Drawing for the job (mm, zero at the part's lowest x, y, z). Give positions to 0.01 mm unless a question says otherwise; leave off trailing zeros. Loops run counter-clockwise (first coordinate to the right, second up) from the corner with the lowest first, then second, coordinate; pieces in that order, holes last. Notation, with made-up numbers: M 14.5,-39 L 54.5,-39 A16 ccw 54.5,-21 Z; hole C 77,12 d3. An arc over 180 degrees is marked long. Answer in a Markdown table with one row per item. Add a question column.
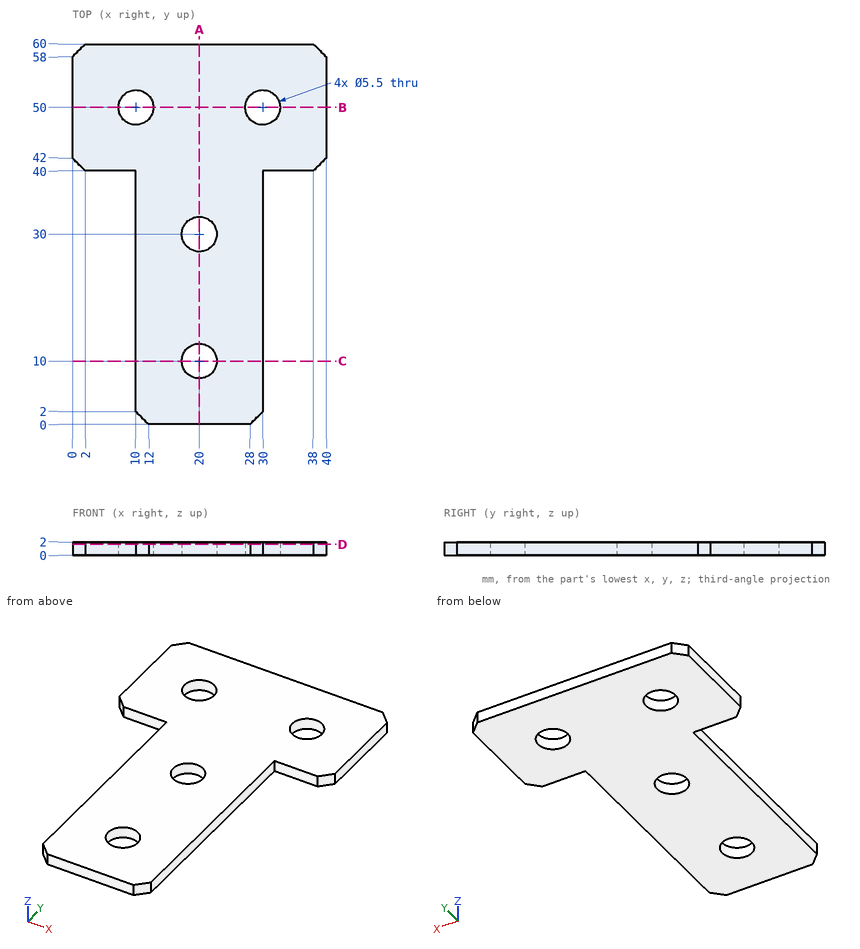
(1) Pin check, flat tips, straight feed: pin 1 (1 mm diameter, centred on x = 35, z = 0.5, fed in from -Y); pin 2 (1 mm diameter, centred on y = 14, z = 1, fed in from +X); pin 3 (3.5 mm diameter, centred on x = 30, y = 50, fed in from +Z); pin 4 (1 mm diameter, centred on x = 29, z = 1.5, fed in from -Y). Stop position of each tip, or through.
(2) Slice it at C-C, the plane y = 10. Give the cut face in (x, z), then the cut area to 3 significant figures.
(3) Slice it at B-B, the plane y = 50. Give the cut face in (x, z).
(4) Slice it at D-D, the plane z = 1.7. Give the cut face in (x, y).
(5) Wall check: line 1 (Y direction, x = 20, z = 1.55); line 2 (X direction, y = 51, z = 0.1); line 3 (X direction, y = 38, z = 0.45). Give the ranges that are in metal, low to high.
(6) Slice it at A-A, the plane x = 20. Give the cut face in (y, z), then the cut area to 3 significant figures.
Solution:
| question | item | result |
|---|---|---|
| 1 | pin 1 | y = 40 |
| 1 | pin 2 | x = 30 |
| 1 | pin 3 | through |
| 1 | pin 4 | y = 0.5 |
| 2 | outline | M 10,0 L 17.25,0 L 17.25,2 L 10,2 Z; M 22.75,0 L 30,0 L 30,2 L 22.75,2 Z |
| 2 | area | 29.0 mm^2 |
| 3 | outline | M 0,0 L 7.25,0 L 7.25,2 L 0,2 Z; M 12.75,0 L 27.25,0 L 27.25,2 L 12.75,2 Z; M 32.75,0 L 40,0 L 40,2 L 32.75,2 Z |
| 4 | outline | M 0,42 L 2,40 L 10,40 L 10,2 L 12,0 L 28,0 L 30,2 L 30,40 L 38,40 L 40,42 L 40,58 L 38,60 L 2,60 L 0,58 Z; hole C 10,50 d5.5; hole C 20,10 d5.5; hole C 20,30 d5.5; hole C 30,50 d5.5 |
| 5 | line 1 | 0 to 7.25, 12.75 to 27.25, 32.75 to 60 |
| 5 | line 2 | 0 to 7.44, 12.56 to 27.44, 32.56 to 40 |
| 5 | line 3 | 10 to 30 |
| 6 | outline | M 0,0 L 7.25,0 L 7.25,2 L 0,2 Z; M 12.75,0 L 27.25,0 L 27.25,2 L 12.75,2 Z; M 32.75,0 L 60,0 L 60,2 L 32.75,2 Z |
| 6 | area | 98.0 mm^2 |
